Can you work these out from the drawing? Everything is in mm from the part's minimum corner. A direction names the side the tool comes from. Give positions to 0.01 mm unless a question says otherwise; leave off trailing zeros. Write each loop counter-clockwise with the first axis right and the second up, starting at its lowest first coordinate (ties: lowest second). Pieces come first, ordered by that corner, then holes. Notation, with made-up numbers: (-3.75, 33.5) -> (29.25, 33.5) arc R17 ccw to (29.25, 54.5) -> close; hole circle Ø2 at (-29.75, 28). An arc over 180 degrees is marked (long way). Return JSON: item names as keys, results as strings.
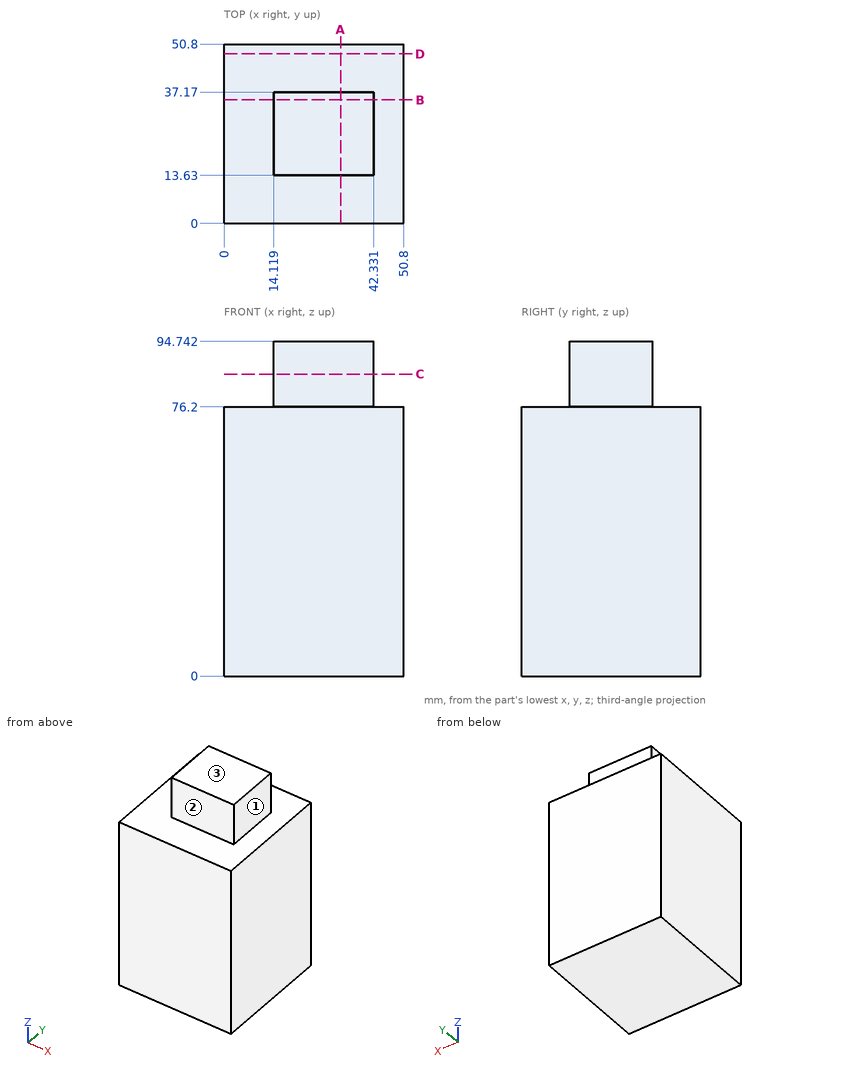
1. If I drill on line 1 (Z direction, x = 2.5, y = 19); line 2 (Y direction, x = 17, z = 87.5); line 3 (X direction, y = 25.5, z = 77.5), over which ranges is the centre line in solid material (lowest first)? Write a range as [from, to].
Taken from the geometry:
{"line 1": "z = [0, 76.2]", "line 2": "y = [13.63, 37.17]", "line 3": "x = [14.12, 42.33]"}
2. Suppose I cut it at B-B, the plane y = 35. List the corners of the cut face in (x, z) for me, and give its area (3 significant figures).
Taken from the geometry:
{"outline": "(0, 0) -> (50.8, 0) -> (50.8, 76.2) -> (42.33, 76.2) -> (42.33, 94.74) -> (14.12, 94.74) -> (14.12, 76.2) -> (0, 76.2) -> close", "area": "4,390 mm²"}
3. Suppose I cut it at A-A, the plane x = 33. List the corners of the cut face in (y, z) for me, and give its area (3 significant figures).
Taken from the geometry:
{"outline": "(0, 0) -> (50.8, 0) -> (50.8, 76.2) -> (37.17, 76.2) -> (37.17, 94.74) -> (13.63, 94.74) -> (13.63, 76.2) -> (0, 76.2) -> close", "area": "4,310 mm²"}
4. Suppose I cut it at C-C, the plane z = 85.5. List the corners of the cut face in (x, y) for me.
Taken from the geometry:
{"outline": "(14.12, 13.63) -> (42.33, 13.63) -> (42.33, 37.17) -> (14.12, 37.17) -> close"}
5. For pin 1 Ø20.5 at (x, z) = (25.5, 89) entering from -Y; pin 2 Ø15 at (y, z) = (27, 88) entering from -X; pin 3 Ø9.5 at (y, z) = (28.5, 88) entering from +X, each with a flat end and sliding along its axis, tell me the tip position at first contact or that it passes through.
Taken from the geometry:
{"pin 1": "stops at y = 13.63", "pin 2": "stops at x = 14.12", "pin 3": "stops at x = 42.33"}
6. Suppose I cut it at D-D, the plane y = 48. List the corners of the cut face in (x, z) for me, and give its area (3 significant figures).
Taken from the geometry:
{"outline": "(0, 0) -> (50.8, 0) -> (50.8, 76.2) -> (0, 76.2) -> close", "area": "3,870 mm²"}
7. Which directions (+Z, -Z, +X, -X, +Y, -Y) give clear straight access to the entire face, cutting with the end or side of a thin tool? Please do the marked faces 1, 2 and 3.
Taken from the geometry:
{"face 1": "+Z, +X, +Y, -Y", "face 2": "+Z, +X, -X, -Y", "face 3": "+Z, +X, -X, +Y, -Y"}
